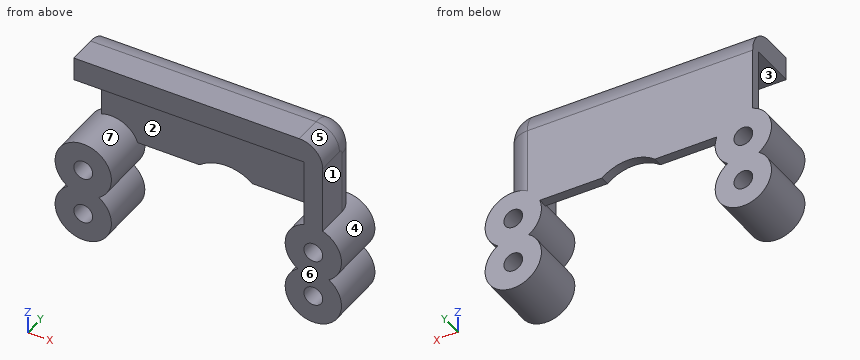
from build123d import *

# Parameters (mm, degrees)
SKETCH1_R             = 2.0000000000000036
SKETCH1_R_2           = 2.0000000000000213
BOSS_EXTRUDE1_DEPTH   = 10
SKETCH1_R_3           = 2.0000000000000013
BOSS_EXTRUDE1_2_DEPTH = 10
SKETCH2_W             = 53.000000000000014
SKETCH2_H             = 22.999999999999996
BOSS_EXTRUDE2_DEPTH   = 2
FILLET1_R             = 6
SKETCH5_R             = 5.999999999999998
SKETCH5_R_2           = 2
SKETCH5_R_3           = 2.0000000000000027
SKETCH5_R_4           = 6.000000000000003
SKETCH5_R_5           = 2.0000000000000067
SKETCH5_R_6           = 5.999999999999995
BOSS_EXTRUDE5_DEPTH   = 2
SKETCH7_R             = 9
CUT_EXTRUDE1_DEPTH    = 2
FILLET2_R             = 5


with BuildPart() as part:
    # Sketch1 → Boss-Extrude1 (new body)
    with BuildSketch(Plane(origin=(0, 0, 0), x_dir=(1, 0, 0), z_dir=(0, 1, 0))):
        with BuildLine():
            ThreePointArc((18.139184902589378, 6.828972817517872), (22.093910791670055, 11.750137196267254), (19.455809692945103, 17.48582706701017))
            ThreePointArc((19.455809692945035, 17.485827067010383), (16.139184902589513, 28.485827067010298), (12.82256011223399, 17.48582706701038))
            ThreePointArc((12.822560112233926, 17.485827067010174), (10.184459013508956, 11.75013719626737), (14.139184902589426, 6.8289728175179505))
            Line((14.139184902589509, 6.828972817517972), (14.139184902589509, -7.5458155744883015))
            Line((14.13918490258951, -7.545815574488302), (-34.86081509741051, -7.545815574488318))
            Line((-34.8608150974105, -7.545815574488319), (-34.8608150974105, -12.514172932989698))
            Line((-34.8608150974105, -12.5141729329897), (18.139184902589513, -12.514172932989684))
            Line((18.139184902589513, -12.514172932989686), (18.139184902589516, 6.828972817517839))
        make_face()
        with Locations(Location((16.139184902589513, 12.485827067010298, 0), (0, 0, 270))):
            Circle(SKETCH1_R, mode=Mode.SUBTRACT)
        with Locations(Location((16.139184902589513, 22.485827067010316, 0), (0, 0, 270))):
            Circle(SKETCH1_R_2, mode=Mode.SUBTRACT)
    extrude(amount=BOSS_EXTRUDE1_DEPTH)



with BuildPart() as body_2:
    # Sketch1 → Boss-Extrude1 2 (new body)
    with BuildSketch(Plane(origin=(0, 0, 0), x_dir=(1, 0, 0), z_dir=(0, 1, 0))):
        with BuildLine():
            ThreePointArc((-36.177439887766084, 17.48582706701017), (-32.860815097410494, 6.485827067010302), (-29.544190307054905, 17.485827067010174))
            ThreePointArc((-29.54419030705497, 17.485827067010383), (-32.86081509741049, 28.485827067010298), (-36.17743988776603, 17.48582706701039))
        make_face()
        with Locations(Location((-32.860815097410494, 12.485827067010298, 0), (0, 0, 270))):
            Circle(SKETCH1_R_3, mode=Mode.SUBTRACT)
        with Locations(Location((-32.860815097410494, 22.485827067010298, 0), (0, 0, 270))):
            Circle(SKETCH1_R, mode=Mode.SUBTRACT)
    extrude(amount=BOSS_EXTRUDE1_2_DEPTH)


with BuildPart() as part_1:
    add(part.part)

    add(body_2.part)  # Boss-Extrude2 merges body 2
    # Sketch2 → Boss-Extrude2 (add)
    with BuildSketch(Plane(origin=(0, 10, 0), x_dir=(1, 0, 0), z_dir=(0, 1, 0))):
        with Locations((-8.360815097410494, -1.0141729329897018)):
            Rectangle(SKETCH2_W, SKETCH2_H)
    extrude(amount=BOSS_EXTRUDE2_DEPTH)

    # Fillet1
    fillet1_edges = [part_1.edges().sort_by_distance(p)[0] for p in [
        (-8.360815097410494, 12, 12.5141729329897),
    ]]
    fillet(fillet1_edges, radius=FILLET1_R)

    # Sketch5 → Boss-Extrude5 (add)
    # profile 1 of 4: a face of its own
    with BuildSketch(Plane(origin=(0, 10, 0), x_dir=(1, 0, 0), z_dir=(0, 1, 0))):
        with Locations((16.139184902589513, 22.485827067010298)):
            Circle(SKETCH5_R)
        with Locations(Location((16.139184902589513, 22.485827067010298, 0), (0, 0, 270))):
            Circle(SKETCH5_R_2, mode=Mode.SUBTRACT)
    # profile 2 of 4: a face of its own
    with BuildSketch(Plane(origin=(0, 10, 0), x_dir=(1, 0, 0), z_dir=(0, 1, 0))):
        with Locations((16.139184902589513, 12.485827067010298)):
            Circle(SKETCH5_R)
        with Locations(Location((16.139184902589513, 12.485827067010298, 0), (0, 0, 270))):
            Circle(SKETCH5_R_3, mode=Mode.SUBTRACT)
    # profile 3 of 4: a face of its own
    with BuildSketch(Plane(origin=(0, 10, 0), x_dir=(1, 0, 0), z_dir=(0, 1, 0))):
        with Locations((-32.860815097410494, 22.485827067010298)):
            Circle(SKETCH5_R_4)
        with Locations(Location((-32.860815097410494, 22.485827067010298, 0), (0, 0, 270))):
            Circle(SKETCH5_R_5, mode=Mode.SUBTRACT)
    # profile 4 of 4: a face of its own
    with BuildSketch(Plane(origin=(0, 10, 0), x_dir=(1, 0, 0), z_dir=(0, 1, 0))):
        with Locations((-32.860815097410494, 12.4858270670103)):
            Circle(SKETCH5_R_6)
        with Locations(Location((-32.860815097410494, 12.4858270670103, 0), (0, 0, 270))):
            Circle(SKETCH5_R_3, mode=Mode.SUBTRACT)
    extrude(amount=BOSS_EXTRUDE5_DEPTH)

    # Sketch7 → Cut-Extrude1 (cut)
    with BuildSketch(Plane(origin=(0, 12, 0), x_dir=(1, 0, 0), z_dir=(0, 1, 0))):
        with Locations((-8.360815097410491, 17.485827067010298)):
            Circle(SKETCH7_R)
    extrude(amount=-CUT_EXTRUDE1_DEPTH, mode=Mode.SUBTRACT)

    # Fillet2
    fillet2_edges = [part_1.edges().sort_by_distance(p)[0] for p in [
        (18.139184902589513, 12, -0.1573999422640835),
        (18.139184902589513, 3.0000000000000004, 12.514172932989688),
        (18.139184902589513, 10.242640687119287, 10.756813620108982),
    ]]
    fillet(fillet2_edges, radius=FILLET2_R)


solid = part_1.part
Source: CAD feature listing. Evaluate the final solid. Frame: model axes, mm. Face numbers are marked on the shaded views. A direction names the side the tool comes from. Round coordinates to 2 decimals unless told otherwise and drop trailing zeros. Loops run counter-clockwise (first coordinate to the right, second up) from the corner with the lowest first, then second, coordinate; pieces in that order, holes last. Notation, with made-up numbers: M 27.5,-25.5 L 42.5,-25.5 A27 cw 42.5,5.5 Z; hole C 7.25,83 d3. An arc over 180 degrees is marked long. Return JSON: item names as keys, results as strings. Group by question number.
1. Section query D-D on z = 4.5. Output: boundary loops of the cut face in (x, y).
2. Material intervals for line 1 along X through (y, z) = (3.25, -22); line 2 along X through (y, z) = (3.5, -21.5); line 3 along X through (y, z) = (3.75, 6), sorted ascending. Write a range as from..to.
3. Section query C-C on z = -13. Output: boundary loops of the cut face in (x, y), and give its area (3 significant figures).
4. Pin query (flat end, axial travel): pin 1 (6 mm diameter, centred on y = 10, z = -3.5, fed in from +X); pin 2 (1 mm diameter, centred on y = 9, z = 3, fed in from +X); pin 3 (1.6 mm diameter, centred on x = 1.5, y = 11.5, fed in from -Z). Return the tip coordinate at first contact, or that it passes through.
5. Section query A-A on y = 2.5. Output: boundary loops of the cut face in (x, z).
6. Reachability of the marked faces 1, 2 and 3 from +Z, -Z, +X, -X, +Y, -Y: full face, straight path, thin tool, end or side. Return the list, or none.
7. Mould query, pull axis Z, two halves, no side actions, for the marked faces 4, 5, 6 and 7. Classes: released by +Z, released by -Z, zero draft, split by the parting line, or undercut.
8. Section query B-B on x = 5. Output: boundary loops of the cut face in (y, z).
Checks:
{
 "1": {"outline": "M -34.86,10 L 14.14,10 L 14.14,0 L 18.14,0 L 18.14,7 A5 ccw 13.14,12 L -34.86,12 Z"},
 "2": {"line 1": "x = -38.84..-34.8, -30.92..-26.88, 10.16..14.2, 18.08..22.12", "line 2": "x = -38.78..-34.6, -31.12..-26.94, 10.22..14.4, 17.88..22.06", "line 3": "x = 14.14..18.14"},
 "3": {"outline": "M -38.84,0 L -34.79,0 L -34.79,12 L -38.84,12 Z; M -30.93,0 L -26.88,0 L -26.88,12 L -30.93,12 Z; M 10.16,0 L 14.21,0 L 14.21,12 L 10.16,12 Z; M 18.07,0 L 22.12,0 L 22.12,12 L 18.07,12 Z", "area": "194 mm²"},
 "4": {"pin 1": "stops at x = 18.14", "pin 2": "stops at x = 17.91", "pin 3": "stops at z = -10.49"},
 "5": {"outline": "M -36.18,-17.49 A6 ccw long -29.54,-17.49 A6 ccw long Z; M -34.86,7.55 L 14.14,7.55 L 14.14,-6.83 A6 ccw 12.82,-17.49 A6 ccw long 19.46,-17.49 A6 ccw 18.14,-6.83 L 18.14,7.51 A5 ccw 13.14,12.51 L -34.86,12.51 Z; hole C -32.86,-22.49 d4; hole C -32.86,-12.49 d4; hole C 16.14,-22.49 d4; hole C 16.14,-12.49 d4"},
 "6": {"face 1": "+Z, +X, +Y, -Y", "face 2": "-Y", "face 3": "-X, -Y"},
 "7": {"face 4": "undercut", "face 5": "released by +Z", "face 6": "zero draft", "face 7": "undercut"},
 "8": {"outline": "M 0,7.55 L 10,7.55 L 10,-10.49 L 12,-10.49 L 12,6.51 A6 ccw 6,12.51 L 0,12.51 Z"}
}
